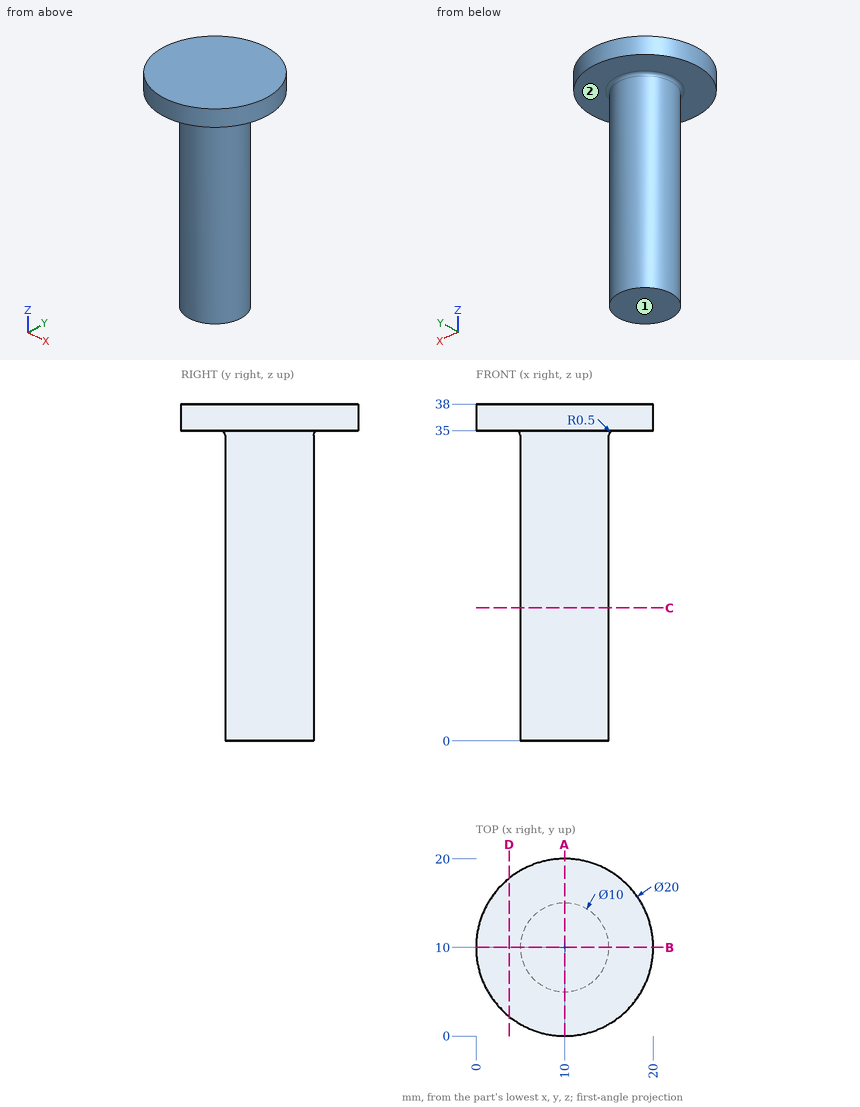
Input: dimensioned drawing with shaded views. Units: mm. Origin: part minimum x, y, z. A direction names the side the tool comes from. Coordinates: 2 decimals unless noted, no trailing zeros. Order: outer loops, then holes, each group sorted by start corner. A loop starts at its lowest first (then second) coordinate and runs counter-clockwise, first axis right, second up.
(1) Section query C-C (z = 15). Return the cut outline in (x, y), plus the area to 3 significant figures.
(2) Material intervals for probe 1 along Z at (x, y) = (1.75, 4.5); probe 2 along X at (y, z) = (14.5, 5), sorted ascending.
(3) Section query D-D (x = 3.75). Return the cut outline in (y, z), plus the area to 3 significant figures.
(4) First-contact query: pin 1 (1 mm diameter, centred on y = 7.5, z = 22.5, fed in from -X); pin 2 (4 mm diameter, centred on x = 16, y = 5, fed in from -Z); pin 3 (6 mm diameter, centred on x = 9, z = 21.5, fed in from -Y); pin 4 (10 mm diameter, centred on x = 14, y = 6, fed in from -Z). Flat tips, straight axial feed; report the tip coordinate or a pass-through.
(5) Section query A-A (x = 10). Return the cut outline in (y, z).
(6) Access query for the marked faces 1 and 2. Directions: +Z, -Z, +X, -X, +Y, -Y. A direction counts if a zero-diameter tool reaches every point of the face in a straight line with its end or side. Return the directions, or none.
Solution:
1. outline: circle Ø10 at (10, 10)
1. area: 78.5 mm2
2. probe 1: z = 35 to 38
2. probe 2: x = 7.82 to 12.18
3. outline: (2.19, 35) - (17.81, 35) - (17.81, 38) - (2.19, 38) - close
3. area: 46.8 mm2
4. pin 1: stops at x = 5.42
4. pin 2: stops at z = 35
4. pin 3: stops at y = 5
4. pin 4: stops at z = 0
5. outline: (0, 35) - (4.5, 35) arc R0.5 cw to (5, 34.5) - (5, 0) - (15, 0) - (15, 34.5) arc R0.5 cw to (15.5, 35) - (20, 35) - (20, 38) - (0, 38) - close
6. face 1: -Z, +X, -X, +Y, -Y
6. face 2: -Z
